Geometry check sheet. Reference: the model listing, model coordinates, mm. A direction names the side the tool comes from. Round coordinates to 2 decimals unless told otherwise and drop trailing zeros. Write each loop counter-clockwise with the first axis right and the second up, starting at its lowest first coordinate (ties: lowest second). Pieces come first, ordered by that corner, then holes.
Item 1: Cross-section at C-C (y = -60). Enter the section's corners in (x, z), then the cut area to 3 significant figures.
Item 2: Cross-section at B-B (x = -3.5). State how many separate pieces and enclosed holes the cut face has, then the cut area to 3 significant figures.
Item 3: Scan lines: probe 1 along X at (y, z) = (-32, 14.5); probe 2 along Y at (x, z) = (-1.5, 18); probe 3 along Y at (x, z) = (-2, 16). Record each from-to range of solid material in increasing order.
Item 4: Depth check by flat-ended pin: P1, Ø6, axis at x = 0.5, y = -44.5, coming from the +Z side; P2, Ø6, axis at x = 0, y = -19.5, coming from the +Z side; P3, Ø8, axis at y = -28.5, z = 18, coming from the -X side. Enter the tip coordinate at first touch or a pass-through.
Item 5: Access from +Z, -Z, +X, -X, +Y, -Y to the whole of each face (thin tool, end or side, straight path). Record for faces 1 (the face through (0, -32, 12.146)), 2 (the face through (-0.542, -34.567, 22.626)).
Item 6: Cross-section at A-A (y = -6.5). Enter the section's corners in (x, z).
from build123d import *

# Parameters (mm, degrees)
F5_R     = 2.5
F6_DEPTH = 25


with BuildPart() as f2:
    # F1 (on Right) → F2 (revolve)
    with BuildSketch(Plane.YZ):
        with BuildLine():
            Line((-65.126866281, 37.146495508), (-55.126866281, 37.146495508))
            ThreePointArc((-55.126866281, 37.146495508), (-55.3055107736, 38.4710826404), (-55.8286787096, 39.7010176944))
            ThreePointArc((-55.8286787096, 39.7010176944), (-61.4514534135, 41.9678510154), (-65.126866281, 37.146495508))
        make_face()
        with BuildLine():
            ThreePointArc((-55.8286787096, 39.7010176944), (-55.3055107736, 38.4710826404), (-55.126866281, 37.146495508))
            Line((-55.126866281, 37.146495508), (-32.126866281, 37.146495508))
            Line((-32.126866281, 37.146495508), (-32.126866281, 42.146495508))
            add(Edge.make_bspline(
                [(-55.8286787096, 39.7010176944), (-52.1369661584, 39.9591630433), (-44.4849831476, 39.7044354809), (-36.3111111426, 42.1526526385), (-32.126866281, 42.146495508)],
                knots=[0, 0, 0, 0, 0.4864401109, 1, 1, 1, 1], degree=3))
        make_face()
    revolve(axis=Axis((0, -43.626866281, 37.146495508), (0, -1, 0)))

    # F3: F2 across face


with BuildPart() as f2_1:
    add(f2.part)
    add(f2.part.mirror(Plane(origin=(0, -32.126866281, 37.146495508), x_dir=(-1, 0, 0), z_dir=(0, 1, 0))))

    # F5 (on plane+point) → F6 (join)
    with BuildSketch(Plane.XY.offset(37.146495508)):
        with Locations((0, -32.126866281)):
            Circle(F5_R)
    extrude(amount=-F6_DEPTH)


solid = f2_1.part
Resolved:
1. outline: circle Ø10 at (0, 37.15)
1. area: 78.5 mm2
2. separate pieces: 3
2. enclosed holes: 0
2. area: 188 mm2
3. probe 1: x = -2.5 to 2.5
3. probe 2: y = -34.13 to -30.13
3. probe 3: y = -33.63 to -30.63
4. P1: stops at z = 40.86
4. P2: stops at z = 40.81
4. P3: stops at x = -2.5
5. face 1: -Z, +X, -X, +Y, -Y
5. face 2: -Z
6. outline: circle Ø8.8 at (0, 37.15)
